from build123d import *

# Parameters (mm, degrees)
SKETCH1_W            = 169
SKETCH1_H            = 84
BOSS_EXTRUDE1_DEPTH  = 5
SKETCH2_W            = 89
SKETCH2_H            = 60
BOSS_EXTRUDE2_DEPTH  = 40
CUT_EXTRUDE1_DEPTH   = 109.212753407
SKETCH4_W            = 13
SKETCH4_H            = 3
CUT_EXTRUDE2_DEPTH   = 120.788355027
SKETCH6_W            = 13
SKETCH6_H            = 27.5
CUT_EXTRUDE5_DEPTH   = 6
FILLET1_R            = 10
FILLET1_OF_MIRROR1_R = 10


with BuildPart() as part:
    # Sketch1 → Boss-Extrude1 (new body)
    with BuildSketch(Plane(origin=(0, 0, 0), x_dir=(1, 0, 0), z_dir=(0, 1, 0))):
        Rectangle(SKETCH1_W, SKETCH1_H)
    extrude(amount=BOSS_EXTRUDE1_DEPTH)

    # Sketch2 → Boss-Extrude2 (add)
    with BuildSketch(Plane(origin=(0, 5, 0), x_dir=(1, 0, 0), z_dir=(0, 1, 0))):
        with Locations((40, 0)):
            Rectangle(SKETCH2_W, SKETCH2_H)
    extrude(amount=BOSS_EXTRUDE2_DEPTH)

    # Sketch3 → Cut-Extrude1 (cut, through all)
    with BuildSketch(Plane.ZY.offset(4.5)):
        with BuildLine():
            Line((-22.5, 45), (22.5, 45))
            ThreePointArc((22.5, 45), (0, 22.5), (-22.5, 45))
        make_face()
    extrude(amount=-CUT_EXTRUDE1_DEPTH, mode=Mode.SUBTRACT)

    # Sketch4 → Cut-Extrude2 (cut, through all)
    with BuildSketch(Plane(origin=(0, 0, -30), x_dir=(-1, 0, 0), z_dir=(0, 0, -1))):
        with Locations((-12, 16)):
            Rectangle(SKETCH4_W, SKETCH4_H)
        with Locations((-68, 16)):
            Rectangle(SKETCH4_W, SKETCH4_H)
    extrude(amount=-CUT_EXTRUDE2_DEPTH, mode=Mode.SUBTRACT)

    # Sketch6 → Cut-Extrude5 (cut)
    with BuildSketch(Plane.XY.offset(30)):
        with Locations((12, 31.25)):
            Rectangle(SKETCH6_W, SKETCH6_H)
        with Locations((68, 31.25)):
            Rectangle(SKETCH6_W, SKETCH6_H)
    cut_extrude5 = extrude(amount=-CUT_EXTRUDE5_DEPTH, mode=Mode.SUBTRACT)

    # Fillet1
    fillet1_edges = [part.edges().sort_by_distance(p)[0] for p in [
        (12, 17.5, 24),
        (68, 17.5, 24),
    ]]
    fillet(fillet1_edges, radius=FILLET1_R)

    # Mirror1: Cut-Extrude5 across plane
    add(cut_extrude5.mirror(Plane.XY), mode=Mode.SUBTRACT)

    # Fillet1 of Mirror1
    fillet1_of_mirror1_edges = [part.edges().sort_by_distance(p)[0] for p in [
        (12, 17.5, -24),
        (68, 17.5, -24),
    ]]
    fillet(fillet1_of_mirror1_edges, radius=FILLET1_OF_MIRROR1_R)


solid = part.part
Here's how the part is built. I have some questions about the finished solid (model axes, mm). A direction names the side the tool comes from. Coordinates: 2 decimals unless noted, no trailing zeros. Order: outer loops, then holes, each group sorted by start corner. A loop starts at its lowest first (then second) coordinate and runs counter-clockwise, first axis right, second up.
Item 1: If we section it at C-C on x = 44: List the corners of the cut face in (y, z) for me, plus the area to 3 significant figures.
Result sheet:
outline: (0, -42) - (5, -42) - (5, -30) - (45, -30) - (45, -22.5) arc R22.5 cw to (45, 22.5) - (45, 30) - (5, 30) - (5, 42) - (0, 42) - close
area: 2,020 mm2
Item 2: If we mould it in two halves opening along Y, with no side actions, what happens to faces 5 (the face through (39, 45, -26)), 6 (the face through (39, 25, -30)), 7 (the face through (68, 17.5, 0))? For each: +Y half, -Y half, draft (parallel to the pull), parting line (faces both ways), or undercut.
Result sheet:
face 5: +Y half
face 6: draft
face 7: undercut
Item 3: If we section it at B-B on z = 0: List the corners of the cut face in (x, y) for me.
Result sheet:
outline: (-84.5, 0) - (84.5, 0) - (84.5, 22.5) - (-4.5, 22.5) - (-4.5, 5) - (-84.5, 5) - close; hole (5.5, 14.5) - (18.5, 14.5) - (18.5, 17.5) - (5.5, 17.5) - close; hole (61.5, 14.5) - (74.5, 14.5) - (74.5, 17.5) - (61.5, 17.5) - close
Item 4: I need wall thicknesses on line 1 (X direction, y = 17, z = 27.5); line 2 (Z direction, x = 77, y = 13.5); line 3 (Y direction, x = -53.5, z = -7). Which ranges of each line are inside material? Lowest first, please.
Result sheet:
line 1: x = -4.5 to 5.5, 18.5 to 61.5, 74.5 to 84.5
line 2: z = -30 to 30
line 3: y = 0 to 5
Item 5: For P1, Ø6.5, axis at x = 12, y = 38, coming from the +Z side; P2, Ø4, axis at x = 68.5, z = -4.5, coming from the +Y side; P3, Ø25, axis at x = -16, z = -7.5, coming from the +Y side, each with a flat end and sliding along its axis, tell me the tip position at first contact or that it passes through.
Result sheet:
P1: stops at z = 24
P2: stops at y = 23.46
P3: stops at y = 26.22
Item 6: If we section it at D-D on y = 19.5: List the corners of the cut face in (x, z) for me.
Result sheet:
outline: (-4.5, -30) - (5.5, -30) - (5.5, -20) - (18.5, -20) - (18.5, -30) - (61.5, -30) - (61.5, -20) - (74.5, -20) - (74.5, -30) - (84.5, -30) - (84.5, 30) - (74.5, 30) - (74.5, 20) - (61.5, 20) - (61.5, 30) - (18.5, 30) - (18.5, 20) - (5.5, 20) - (5.5, 30) - (-4.5, 30) - close
Item 7: For faces 1 (the face through (68, 36, -24)), 2 (the face through (68.09, 20.51, -21.15)), 3 (the face through (68.09, 20.35, 20.99)), 4 (the face through (39, 25, 30)), which set-ups out of +Z, -Z, +X, -X, +Y, -Y let a thin tool reach every point of the face, with its end or its side?
Result sheet:
face 1: -Z, +Y
face 2: -Z
face 3: +Z
face 4: +Z, +X, -X, +Y
Item 8: If we section it at A-A on y = 41: List the corners of the cut face in (x, z) for me.
Result sheet:
outline: (-4.5, -30) - (5.5, -30) - (5.5, -24) - (18.5, -24) - (18.5, -30) - (61.5, -30) - (61.5, -24) - (74.5, -24) - (74.5, -30) - (84.5, -30) - (84.5, -22.14) - (-4.5, -22.14) - close; (-4.5, 22.14) - (84.5, 22.14) - (84.5, 30) - (74.5, 30) - (74.5, 24) - (61.5, 24) - (61.5, 30) - (18.5, 30) - (18.5, 24) - (5.5, 24) - (5.5, 30) - (-4.5, 30) - close
